Autodesk Inventor part; units mm, degrees
ref_plane "YZ Plane" through (0, 0, 0) normal (1, 0, 0) x (0, 1, 0)
ref_plane "XZ Plane" through (0, 0, 0) normal (0, 1, 0) x (-1, 0, 0)
ref_plane "XY Plane" through (0, 0, 0) normal (0, 0, 1) x (1, 0, 0)
sketch "Sketch1" plane through (0, 0, 0) normal (1, 0, 0) x (0, 1, 0)
  line L0 (0, 0) -> (16, 0)
  line L1 (16, 0) -> (16, -24)
  line L2 (16, -24) -> (0, -24)
  line L3 (0, -24) -> (0, 0)
  dimension "d0" = 16
  dimension "d1" = 24
extrude "Extrusion1" add sketch "Sketch1" along normal blind 2
sketch "Sketch2" plane through (2, 0, 0) normal (1, 0, 0) x (0, 0, -1)
  line L0 (24, 16) -> (0, 16)
  line L1 (0, 16) -> (24, 16)
  line L2 (24, 16) -> (24, 14)
  line L3 (24, 14) -> (0, 14)
  line L4 (0, 14) -> (0, 16)
  line L5 (0, 16) -> (0, 0)
  line L6 (0, 0) -> (24, 0)
  line L7 (24, 0) -> (24, 2)
  line L8 (24, 2) -> (0, 2)
  line L9 (0, 2) -> (0, 0)
  dimension "d4" = 24
  dimension "d5" = 2
  dimension "d6" = 24
  dimension "d7" = 2
extrude "Extrusion2" add sketch "Sketch2" along normal blind 11
sketch "Sketch3" plane through (0, 0, -24) normal (0, -1, 0) x (1, 0, 0)
  line L0 (13, 24) -> (11, 24)
  line L1 (11, 24) -> (11, 0)
  line L2 (11, 0) -> (13, 0)
  line L3 (13, 0) -> (13, 24)
  point P0 (0, 24)
  dimension "d10" = 2
  dimension "d11" = 24
extrude "Extrusion3" add sketch "Sketch3" along normal blind 10
sketch "Sketch4" plane through (0, 16, 0) normal (0, 1, 0) x (1, 0, 0)
  line L0 (13, 24) -> (13, 0)
  line L1 (13, 24) -> (11, 24)
  line L2 (11, 24) -> (11, 0)
  line L3 (11, 0) -> (13, 0)
  line L4 (13, 0) -> (13, 24)
  point P0 (0, 0)
  point P1 (13, 0)
  dimension "d14" = 2
  dimension "d15" = 24
extrude "Extrusion4" add sketch "Sketch4" along normal blind 10
sketch "Sketch5" plane through (13, 0, 0) normal (1, 0, 0) x (0, 0, -1)
  line L0 (0, 0) -> (0, -5)
  line L1 (0, 2) -> (0, -10)
  line L2 (0, -5) -> (12, -5)
  line L3 (24, 0) -> (24, -10)
  circle A0 centre (12, -5) radius 1.25
  line L4 (0, 14) -> (24, 14)
  line L5 (0, 14) -> (0, 21)
  line L6 (0, 14) -> (0, 26)
  line L7 (0, 21) -> (12, 21)
  circle A1 centre (12, 21) radius 1.25
  dimension "d18" = 5
  dimension "d19" = 12
  dimension "d20" = 2.5
  dimension "d21" = 7
  dimension "d22" = 12
  dimension "d23" = 2.5
extrude "Extrusion5" cut sketch "Sketch5" against normal blind 10
sketch "Sketch7" plane through (0, 0, 0) normal (-1, 0, 0) x (0, 0, 1)
  line L0 (-20, 5) -> (-8, 5)
  line L1 (-8, 5) -> (-8, 11)
  line L2 (-8, 11) -> (-20, 11)
  line L3 (-20, 11) -> (-20, 5)
  line L4 (-24, 0) -> (-24, 16)
  point P0 (0, 0)
  dimension "d26" = 6
  dimension "d27" = 12
  dimension "d28" = 5
  dimension "d29" = 4
extrude "Extrusion6" cut sketch "Sketch7" against normal blind 10
sketch "Sketch8" plane through (0, 0, 0) normal (0, 0, 1) x (1, 0, 0)
  line L0 (11, -10) -> (13, -10)
  line L1 (11, -10) -> (13, -10)
  line L2 (13, 2) -> (13, -10)
  line L3 (13, -10) -> (13, 2)
  line L4 (2, 2) -> (13, 2)
  line L5 (13, 2) -> (2, 2)
  line L6 (2, 14) -> (2, 2)
  line L7 (2, 2) -> (2, 14)
  line L8 (13, 14) -> (13, 26)
  line L9 (2, 14) -> (13, 14)
  line L10 (13, 14) -> (13, 26)
  line L11 (11, 16) -> (11, 26)
  line L12 (13, 26) -> (11, 26)
  line L13 (11, 26) -> (11, 16)
  line L14 (11, 16) -> (0, 16)
  line L15 (0, 0) -> (11, 0)
  line L16 (0, 16) -> (0, 0)
  line L17 (0, 0) -> (11, 0)
  line L18 (11, 0) -> (11, -10)
  line L19 (11, 0) -> (11, -10)
extrude "Extrusion7" cut sketch "Sketch8" against normal blind 4
chamfer "Chamfer1" distance 2 angle 45 2 edges at (12, -10, -24) (12, 26, -24)
chamfer "Chamfer2" distance 2 angle 45 2 edges at (12, -10, -4) (12, 26, -4)
properties part number "houder motor"
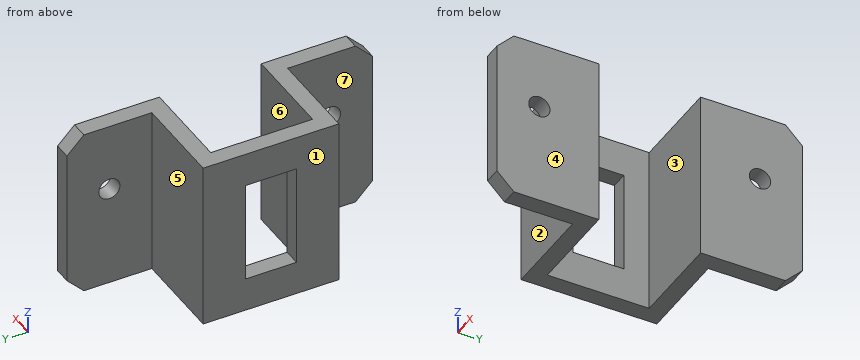
Read the model definition and answer for the solid it produces. Units are mm, in the model's axes. Face numbers are marked on the shaded views. A direction names the side the tool comes from. Give positions to 0.01 mm unless a question says otherwise; leave off trailing zeros. Write each loop counter-clockwise with the first axis right and the second up, starting at its lowest first coordinate (ties: lowest second). Pieces come first, ordered by that corner, then holes. Notation, with made-up numbers: (-0.5, 6) -> (33.5, 6) arc R15 ccw to (33.5, 23) -> close; hole circle Ø11 at (68.25, 26). An arc over 180 degrees is marked (long way). Answer as a JSON object with one key per item and string values.
1) Section A-A on x = 11.5 is taken. Write down the section's boundary in (y, z), then the cut area to 3 significant figures.
Findings below:
{"outline": "(-10, -22) -> (-8, -24) -> (2, -24) -> (2, -4) -> (-8, -4) -> (-10, -6) -> close; (14, -24) -> (24, -24) -> (26, -22) -> (26, -6) -> (24, -4) -> (14, -4) -> close; hole circle Ø2.5 at (-5, -12); hole circle Ø2.5 at (21, -12)", "area": "462 mm^2"}
2) A tool of negligible diameter and unlimited length cuts with its end or side. For the marked faces 4, 5, 6 and 7, from which of +Z, -Z, +X, -X, +Y, -Y can it reach the whole face along a straight path? Write none if from no direction.
Findings below:
{"face 4": "+Z, -Z, +X, +Y, -Y", "face 5": "+Z, -Z, -X, +Y", "face 6": "+Z, -Z, +X", "face 7": "+Z, -Z, -X, -Y"}
3) Section D-D on z = -14.25 is taken. Write down the section's boundary in (x, y), then the cut area to 3 significant figures.
Findings below:
{"outline": "(0, 0) -> (11, 0) -> (11, -10) -> (13, -10) -> (13, 2) -> (2, 2) -> (2, 5) -> (0, 5) -> close; (0, 11) -> (2, 11) -> (2, 14) -> (13, 14) -> (13, 26) -> (11, 26) -> (11, 16) -> (0, 16) -> close", "area": "104 mm^2"}
4) Straight lines are drawn through the part: probe 1 along Y at (x, z) = (12.2, -12); probe 2 along Y at (x, z) = (10.5, -16.75); probe 3 along Y at (x, z) = (12, -21). For each, find the intervals that lie inside material, in ascending order. Write a range as from..to.
Findings below:
{"probe 1": "y = -10..-6.25, -3.75..2, 14..19.75, 22.25..26", "probe 2": "y = 0..2, 14..16", "probe 3": "y = -10..2, 14..26"}
5) Section B-B on z = -12 is taken. Write down the section's boundary in (x, y).
Findings below:
{"outline": "(0, 0) -> (11, 0) -> (11, -3.75) -> (13, -3.75) -> (13, 2) -> (2, 2) -> (2, 5) -> (0, 5) -> close; (0, 11) -> (2, 11) -> (2, 14) -> (13, 14) -> (13, 19.75) -> (11, 19.75) -> (11, 16) -> (0, 16) -> close; (11, -10) -> (13, -10) -> (13, -6.25) -> (11, -6.25) -> close; (11, 22.25) -> (13, 22.25) -> (13, 26) -> (11, 26) -> close"}
6) Flat-ended cylindrical pins translate along their axes: pin 1 Ø9.5 at (y, z) = (8.5, -17.5) entering from +X; pin 2 Ø5 at (y, z) = (19.5, -10) entering from -X; pin 3 Ø5.5 at (x, z) = (4.5, -11.5) entering from +Y; pin 4 Ø2 at (y, z) = (-5, -12) entering from +X. Find the tip coordinate at first contact, or state that the pin passes through.
Findings below:
{"pin 1": "stops at x = 2", "pin 2": "stops at x = 11", "pin 3": "stops at y = 16", "pin 4": "passes through"}
7) For a pull along Y with two mould halves and no side action, classify the marked faces 1, 2 and 3 as pulls with the +Y half, pulls with the -Y half, needs draft (parallel to the pull), parting line crosses it, or undercut.
Findings below:
{"face 1": "needs draft", "face 2": "pulls with the -Y half", "face 3": "undercut"}
8) Section C-C on y = 7 is taken. Write down the section's boundary in (x, z), then the cut area to 3 significant figures.
Findings below:
{"outline": "(0, -24) -> (2, -24) -> (2, -20) -> (0, -20) -> close; (0, -8) -> (2, -8) -> (2, -4) -> (0, -4) -> close", "area": "16.0 mm^2"}
